Here's the drawing with two shaded views (mm, measured from the low corner). I have some questions. A direction names the side the tool comes from. Coordinates: 2 decimals unless noted, no trailing zeros. Loops run counter-clockwise (first coordinate to the right, second up) from the corner with the lowest first, then second, coordinate; pieces in that order, holes last. Notation, with made-up numbers: (-14, 32) - (27, 32) arc R23 ccw to (27, 56) - close; hole circle Ø11 at (26.5, -16.5). An arc over 180 degrees is marked (long way). One line per item, written item: value. Start each with the question number.
(1) If we section it at A-A on z = 15.25: Write out the boundary of the cut face in (x, y).
(2) If we mould it in two halves opening along Z, with no side actions, what happens to the marked faces 1, 2 and 3? For each: pulls with the +Z half, pulls with the -Z half, needs draft (parallel to the pull), parting line crosses it, or undercut.
(3) If I drill on line 1 along Z through (x, y) = (4, 15.25); line 2 along Z through (x, y) = (11, 15), over which ranges is the centre line in solid material (lowest first)? Write a range as from..to.
(4) If we section it at B-B on y = 13.5: Write out the boundary of the cut face in (x, z), then the cut area to 3 significant figures.
(5) If we section it at C-C on x = 6.25: Write out the boundary of the cut face in (y, z), then the cut area to 3 significant figures.
(6) I'm going to push flat-ended pins straight in: P1, Ø14.5, axis at y = 15.25, z = 15.25, coming from the -X side; P2, Ø1, axis at x = 12, y = 22, coming from the +Z side; P3, Ø4, axis at y = 26, z = 18.5, coming from the -X side; P4, Ø1.5, axis at x = 1.5, z = 24, coming from the +Y side. Where does each tip first touch, or does it pass through?
(7) If we section it at D-D on z = 29: Write out the boundary of the cut face in (x, y).
(8) On a 3-axis mill with a long thin cutter (end or side, diameter ignored), from which of +Z, -Z, +X, -X, +Y, -Y can I reach the whole of each face in a straight line? I mean the marked faces 4, 5 and 6. Say none if no direction works.
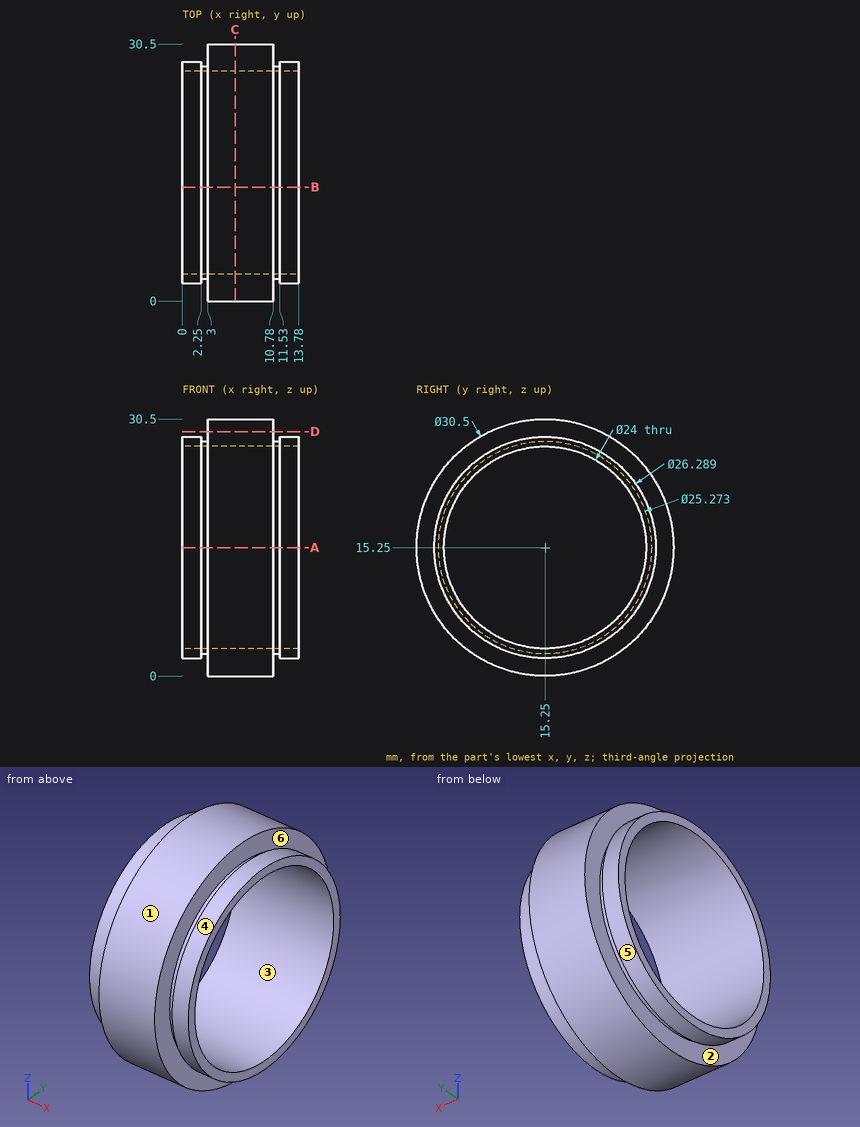
Values:
1. outline: (0, 2.11) - (2.25, 2.11) - (2.25, 2.61) - (3, 2.61) - (3, 0) - (10.78, 0) - (10.78, 2.61) - (11.53, 2.61) - (11.53, 2.11) - (13.78, 2.11) - (13.78, 3.25) - (0, 3.25) - close; (0, 27.25) - (13.78, 27.25) - (13.78, 28.39) - (11.53, 28.39) - (11.53, 27.89) - (10.78, 27.89) - (10.78, 30.5) - (3, 30.5) - (3, 27.89) - (2.25, 27.89) - (2.25, 28.39) - (0, 28.39) - close
2. face 1: parting line crosses it
2. face 2: needs draft
2. face 3: undercut
3. line 1: z = 0..3.25, 27.25..30.5
3. line 2: z = 2.62..3.25, 27.25..27.88
4. outline: (0, 2.22) - (2.25, 2.22) - (2.25, 2.74) - (3, 2.74) - (3, 0.1) - (10.78, 0.1) - (10.78, 2.74) - (11.53, 2.74) - (11.53, 2.22) - (13.78, 2.22) - (13.78, 3.38) - (0, 3.38) - close; (0, 27.12) - (13.78, 27.12) - (13.78, 28.28) - (11.53, 28.28) - (11.53, 27.76) - (10.78, 27.76) - (10.78, 30.4) - (3, 30.4) - (3, 27.76) - (2.25, 27.76) - (2.25, 28.28) - (0, 28.28) - close
4. area: 63.3 mm2
5. outline: circle Ø30.5 at (15.25, 15.25); hole circle Ø24 at (15.25, 15.25)
5. area: 278 mm2
6. P1: passes through
6. P2: stops at z = 26.81
6. P3: stops at x = 0
6. P4: stops at y = 25.68
7. outline: (3, 8.65) - (10.78, 8.65) - (10.78, 21.85) - (3, 21.85) - close
8. face 4: +X
8. face 5: -X
8. face 6: none
